```python
from build123d import *

# Parameters (mm, degrees)
BOX002_W          = 30
BOX002_H          = 10
BOX002_DEPTH      = 13
BOX001_W          = 30
BOX001_H          = 10
BOX001_DEPTH      = 17
CYLINDER_R        = 10.5
CYLINDER_DEPTH    = 20
CYLINDER001_R     = 20
CYLINDER001_DEPTH = 20
CYLINDER003_R     = 10.25
CYLINDER003_DEPTH = 17
CYLINDER002_R     = 11.5
CYLINDER002_DEPTH = 13
BOX_W             = 26
BOX_H             = 15
BOX_DEPTH         = 17
FILLET_R          = 0.4
FILLET001_R       = 0.55
FILLET002_R       = 0.55


with BuildPart() as cube002:
    # Box002 → Box002 (new body)
    with BuildSketch(Plane(origin=(-15, -5, 0), x_dir=(1, 0, 0), z_dir=(0, 0, 1))):
        with Locations((15, 5)):
            Rectangle(BOX002_W, BOX002_H)
    extrude(amount=BOX002_DEPTH)


with BuildPart() as cube001:
    # Box001 → Box001 (new body)
    with BuildSketch(Plane(origin=(-15, -8, 0), x_dir=(1, 0, 0), z_dir=(0, 0, 1))):
        with Locations((15, 5)):
            Rectangle(BOX001_W, BOX001_H)
    extrude(amount=BOX001_DEPTH)


with BuildPart() as obj1:
    # Cylinder → Cylinder (new body)
    with BuildSketch(Plane.XY):
        Circle(CYLINDER_R)
    extrude(amount=CYLINDER_DEPTH)


with BuildPart() as cut:
    # Cylinder001 → Cylinder001 (new body)
    with BuildSketch(Plane.XY):
        Circle(CYLINDER001_R)
    extrude(amount=CYLINDER001_DEPTH)

    # Cut: cut obj1
    add(obj1.part, mode=Mode.SUBTRACT)


with BuildPart() as cylinder003:
    # Cylinder003 → Cylinder003 (new body)
    with BuildSketch(Plane(origin=(0, -3, 0), x_dir=(1, 0, 0), z_dir=(0, 0, 1))):
        Circle(CYLINDER003_R)
    extrude(amount=CYLINDER003_DEPTH)


with BuildPart() as fusion:
    # Cylinder002 → Cylinder002 (new body)
    with BuildSketch(Plane(origin=(0, -3, 0), x_dir=(1, 0, 0), z_dir=(0, 0, 1))):
        Circle(CYLINDER002_R)
    extrude(amount=CYLINDER002_DEPTH)

    # Fusion: union Cylinder003
    add(cylinder003.part)


with BuildPart() as fillet002:
    # Box → Box (new body)
    with BuildSketch(Plane(origin=(-13, -2, 0), x_dir=(1, 0, 0), z_dir=(0, 0, 1))):
        with Locations((13, 7.5)):
            Rectangle(BOX_W, BOX_H)
    extrude(amount=BOX_DEPTH)

    # Cut001: cut Fusion
    add(fusion.part, mode=Mode.SUBTRACT)

    # Cut002: cut Cut
    add(cut.part, mode=Mode.SUBTRACT)

    # Cut002003: cut Cube001
    add(cube001.part, mode=Mode.SUBTRACT)

    # Cut002004: cut Cube002
    add(cube002.part, mode=Mode.SUBTRACT)

    # Fillet
    fillet_edges = [fillet002.edges().sort_by_distance(p)[0] for p in [
        (-9.233093, 5, 6.5),
        (9.233093, 5, 6.5),
        (-8.261356, 5, 6.5),
        (8.261356, 5, 6.5),
    ]]
    fillet(fillet_edges, radius=FILLET_R)

    # Fillet001
    fillet001_edges = [fillet002.edges().sort_by_distance(p)[0] for p in [
        (10.307764, 2, 15),
        (8.947765, 2, 15),
    ]]
    fillet(fillet001_edges, radius=FILLET001_R)

    # Fillet002
    fillet002_edges = [fillet002.edges().sort_by_distance(p)[0] for p in [
        (-10.307764, 2, 15),
        (-8.947765, 2, 15),
    ]]
    fillet(fillet002_edges, radius=FILLET002_R)


solid = fillet002.part
```
Verification items for the finished model (mm, model axes). A direction names the side the tool comes from. Coordinates: 2 decimals unless noted, no trailing zeros. Order: outer loops, then holes, each group sorted by start corner. A loop starts at its lowest first (then second) coordinate and runs counter-clockwise, first axis right, second up. Notation, with made-up numbers: (77.25, -3) -> (112.25, -3) arc R17 cw to (112.25, 5) -> close; hole circle Ø7 at (81, -1.5). An arc over 180 degrees is marked (long way). Answer as CSV lines item,"result". Start each with the question number.
1) Set-up check for faces 5 (the face through (0, 9, 0)), 6 (the face through (0.1, 8.5, 6.4)): record each of +Z, -Z, +X, -X, +Y, -Y from which the full face is reachable in a straight line by a thin tool's end or side.
2) Cross-section at B-B, the plane z = 14. Record the boundary of the cut face in (x, y).
3) Cross-section at C-C, the plane x = 4.25. Record the boundary of the cut face in (y, z).
4) Cross-section at A-A, the plane y = 3. Record the boundary of the cut face in (x, z).
5) Release check for a two-part mould opening along X. For faces 1 (the face through (0, 8, 17)), 2 (the face through (0.2, 10.5, 8.4)), 3 (the face through (0, 7.4, 13)), 4 (the face through (0.15, 7.25, 14.97)) record: released by +X, released by -X, zero draft, split by the parting line, or undercut.
6) Cross-section at D-D, the plane y = 6.75. Record the boundary of the cut face in (x, z), then the cut area to 3 significant figures.
7) Material ranges on L1, parallel to Y at x = 0, z = 2.5; L2, parallel to Y at x = -0.25, z = 13.5; L3, parallel to Z at x = -4.25, y = 7.5, recorded low to high. Write a range as [from, to].
8) Gauge pin test, flat ends, axial feed: pin 1 Ø8 at (x, z) = (-5, 12) entering from +Y; pin 2 Ø1.5 at (y, z) = (7.5, 11) entering from -X; pin 3 Ø1.5 at (x, z) = (-4, 10) entering from +Y; pin 4 Ø2 at (x, y) = (2, 6) entering from -Z. Record the tip position at first contact, or that the pin passes through.
Conclusion:
1,face 5,"-Z, +X, -X, +Y, -Y"
1,face 6,"-Z, -Y"
2,outline,"(-10.15, 2.69) arc R0.55 ccw to (-9.62, 2) -> (-9.26, 2) arc R0.55 ccw to (-8.79, 2.27) arc R10.25 cw to (8.79, 2.27) arc R0.55 ccw to (9.26, 2) -> (9.62, 2) arc R0.55 ccw to (10.15, 2.69) arc R10.5 ccw to start"
3,outline,"(6.33, 13) -> (7.69, 13) -> (7.69, 0) -> (9.6, 0) -> (9.6, 17) -> (6.33, 17) -> close"
4,outline,"(-10.06, 13) -> (-8.31, 13) -> (-8.31, 17) -> (-10.06, 17) -> close; (8.31, 13) -> (10.06, 13) -> (10.06, 17) -> (8.31, 17) -> close"
5,face 1,"zero draft"
5,face 2,"split by the parting line"
5,face 3,"undercut"
5,face 4,"undercut"
6,outline,"(-8.04, 0) -> (-6.1, 0) -> (-6.1, 13) -> (-3.16, 13) -> (-3.16, 17) -> (-8.04, 17) -> close; (3.16, 13) -> (6.1, 13) -> (6.1, 0) -> (8.04, 0) -> (8.04, 17) -> (3.16, 17) -> close"
6,area,"89.6 mm²"
7,L1,"y = [8.5, 10.5]"
7,L2,"y = [7.25, 10.5]"
7,L3,"z = [13, 17]"
8,pin 1,"stops at y = 10.45"
8,pin 2,"stops at x = -8.04"
8,pin 3,"stops at y = 9.98"
8,pin 4,"passes through"
